Input: part model. Units: mm. Frame: model coordinates. A direction names the side the tool comes from. Coordinates: 2 decimals unless noted, no trailing zeros. Loops run counter-clockwise (first coordinate to the right, second up) from the corner with the lowest first, then second, coordinate; pieces in that order, holes last.
(1) Line query: L1, parallel to X at y = 36, z = -5.5; L2, parallel to Z at x = 36, y = 34; L3, parallel to Y at x = 35, z = -28. Output: solid intervals per line, ascending.
(2) Section C-C, the plane y = 56. Return loops of the section in (x, z), then the cut area to 3 significant figures.
(3) Mould query, pull axis Z, two halves, no side actions, for faces 4 (the face through (21, 0, -21)), 5 (the face through (11.241, 40.986, -15.924)), 6 (the face through (5.57, 35.07, -7)). Classes: released by +Z, released by -Z, zero draft, split by the parting line, or undercut.
(4) Section B-B, the plane z = -21. Return loops of the section in (x, y).
(5) Set-up query: faces 1 (the face through (21.971, 52.846, -23.304)), 2 (the face through (20.308, 52.846, -19.124)), 3 (the face through (42, 20, -21)). Return all of +Z, -Z, +X, -X, +Y, -Y with unobstructed straight access to the full face (end or side cutting, diameter ignored); none if empty.
(6) Section D-D, the plane x = 8. Return loops of the section in (y, z).
(7) Section A-A, the plane x = 36.5. Return loops of the section in (y, z).
(8) Contact query for flat-ended pins moving along their axis: P1, Ø4, axis at x = 36.5, z = -5.5, coming from the +Y side; P2, Ø0.9, axis at x = 5.5, z = -5.5, coming from the +Y side; P3, Ø8, axis at x = 30.5, z = -27.5, coming from the +Y side. Output: stop coordinate, or through.
```python
from build123d import *

# Parameters (mm, degrees)
SKETCH1_W               = 42
SKETCH1_H               = 42
BOSS_EXTRUDE1_DEPTH     = 40
CHAMFER1_SIZE           = 3
SKETCH2_R               = 11
BOSS_EXTRUDE2_DEPTH     = 2
SKETCH3_R               = 2.5
BOSS_EXTRUDE3_DEPTH     = 22
CUT_EXTRUDE1_DEPTH      = 88.315519812
CUT_EXTRUDE1_DEPTH_BACK = 22
SKETCH5_R               = 1.5
CUT_EXTRUDE2_DEPTH      = 10


with BuildPart() as part:
    # Sketch1 → Boss-Extrude1 (new body)
    with BuildSketch(Plane(origin=(0, 0, 0), x_dir=(1, 0, 0), z_dir=(0, 1, 0))):
        with Locations((21, 21)):
            Rectangle(SKETCH1_W, SKETCH1_H)
    extrude(amount=BOSS_EXTRUDE1_DEPTH)

    # Chamfer1
    chamfer1_edges = [part.edges().sort_by_distance(p)[0] for p in [
        (0, 20, -42),
        (42, 20, -42),
        (42, 20, 0),
        (0, 20, 0),
    ]]
    chamfer(chamfer1_edges, length=CHAMFER1_SIZE)

    # Sketch2 → Boss-Extrude2 (add)
    with BuildSketch(Plane(origin=(0, 40, 0), x_dir=(1, 0, 0), z_dir=(0, 1, 0))):
        with Locations(Location((21, 21, 0), (0, 0, 270))):
            Circle(SKETCH2_R)
    extrude(amount=BOSS_EXTRUDE2_DEPTH)

    # Sketch3 → Boss-Extrude3 (add)
    with BuildSketch(Plane(origin=(0, 42, 0), x_dir=(1, 0, 0), z_dir=(0, 1, 0))):
        with Locations(Location((21, 21, 0), (0, 0, 270))):
            Circle(SKETCH3_R)
    extrude(amount=BOSS_EXTRUDE3_DEPTH)

    # Sketch4 → Cut-Extrude1 (cut, two sides: drawn at the far end of the back side and taken through both)
    with BuildSketch(Plane(origin=(0, 64, 0), x_dir=(1, 0, 0), z_dir=(0, 1, 0)).offset(-CUT_EXTRUDE1_DEPTH_BACK)):
        Polygon((91.105119446, -7.851665626), (21.689600393, 18.596991199), (18.886199661, 19.665141159), (-50.529319392, 46.113797983), (-103.426633041, -92.717240123), (38.207805797, -146.682703732), align=None)
    extrude(amount=CUT_EXTRUDE1_DEPTH + CUT_EXTRUDE1_DEPTH_BACK, mode=Mode.SUBTRACT)

    # Sketch5 → Cut-Extrude2 (cut)
    with BuildSketch(Plane(origin=(0, 40, 0), x_dir=(1, 0, 0), z_dir=(0, 1, 0))):
        with Locations(Location((36.5, 36.5, 0), (0, 0, 270))):
            Circle(SKETCH5_R)
        with Locations(Location((36.5, 5.5, 0), (0, 0, 270))):
            Circle(SKETCH5_R)
        with Locations(Location((5.5, 5.5, 0), (0, 0, 270))):
            Circle(SKETCH5_R)
        with Locations(Location((5.5, 36.5, 0), (0, 0, 270))):
            Circle(SKETCH5_R)
    extrude(amount=-CUT_EXTRUDE2_DEPTH, mode=Mode.SUBTRACT)


solid = part.part
```
Report:
1. L1: x = 0 to 4, 7 to 35, 38 to 42
1. L2: z = -42 to -37.91, -35.09 to -6.91, -4.09 to 0
1. L3: y = 0 to 40
2. outline: (18.89, -19.67) arc R2.5 ccw (long way) to (21.69, -18.6) - close
2. area: 18.6 mm2
3. face 4: zero draft
3. face 5: split by the parting line
3. face 6: undercut
4. outline: (0, 0) - (42, 0) - (42, 40) - (32, 40) - (32, 42) - (23.5, 42) - (23.5, 64) - (18.5, 64) - (18.5, 42) - (10, 42) - (10, 40) - (0, 40) - close
5. face 1: +Y
5. face 2: +Z, -X, +Y
5. face 3: +Z, -Z, +X, +Y, -Y
6. outline: (0, -42) - (40, -42) - (40, 0) - (0, 0) - close
7. outline: (0, -42) - (40, -42) - (40, -38) - (30, -38) - (30, -35) - (40, -35) - (40, -7) - (30, -7) - (30, -4) - (40, -4) - (40, 0) - (0, 0) - close
8. P1: stops at y = 40
8. P2: stops at y = 30
8. P3: stops at y = 42
